Build history of the part. All positions in model axes, mm. Give positions to 0.01 mm unless a question says otherwise; leave off trailing zeros. Loops run counter-clockwise (first coordinate to the right, second up) from the corner with the lowest first, then second, coordinate; pieces in that order, holes last. Notation, with made-up numbers: M 88.25,12.5 L 123.25,12.5 A16 ccw 123.25,19.5 Z; hole C 0,66.25 d1. An arc over 180 degrees is marked long. Answer as a JSON object with one key per item and string values. Group by question number.
1. Slice it at A-A (x = 32.5). List the corners of the cut face in (y, z), then the cut area to 3 significant figures.
2. Mould opens along Z. For faces 1 (the face through (-10, 35, 20)), 2 (the face through (-0.462, 51.005, 19.493)), 3 (the face through (34.415, 35.496, 5.381)) say: released by +Z, released by -Z, zero draft, split by the parting line, or undercut.
3. Slice it at B-B (z = 11.25). Give the number of separate pieces and of enclosed holes in the cut face, then the cut area to 3 significant figures.
4. Drill centre lines: line 1 along X through (y, z) = (17, 11.25); line 2 along X through (y, z) = (7.5, 7.5); line 3 along Z through (x, y) = (-32.5, 27). Where is each one in solid material? Low to high. Write a range as [from, to].
5. Drop flat-ended pins along their axis: pin 1 Ø8 at (x, z) = (-70.5, 11) entering from -Y; pin 2 Ø3 at (x, z) = (-40, 7.5) entering from -Y; pin 3 Ø10 at (x, z) = (-55, 13) entering from -Y; pin 4 Ø6 at (x, z) = (32.5, 10) entering from -Y. Give the stop position or say it passes through.
from build123d import *

# Parameters (mm, degrees)
SKETCH1_W           = 86
SKETCH1_H           = 72
BOSS_EXTRUDE1_DEPTH = 20
SKETCH2_R           = 5
CUT_EXTRUDE1_DEPTH  = 87.214847909
FILLET1_R           = 0.5
FILLET2_R           = 0.5
SKETCH6_W           = 20
SKETCH6_H           = 72
BOSS_EXTRUDE2_DEPTH = 53
CAVITY1_OUTLINE_R   = 5
CAVITY1_DEPTH       = 20
CUT_EXTRUDE2_DEPTH  = 122.65525076


# Read off the part's stored shape, not the designer's step: Cavity1
with BuildPart() as part:
    # Sketch1 → Boss-Extrude1 (new body)
    with BuildSketch(Plane.XY):
        with Locations((0, 36)):
            Rectangle(SKETCH1_W, SKETCH1_H)
    extrude(amount=BOSS_EXTRUDE1_DEPTH)

    # Sketch2 → Cut-Extrude1 (cut, through all)
    with BuildSketch(Plane(origin=(0, 0, 0), x_dir=(1, 0, 0), z_dir=(0, 1, 0))):
        with Locations(Location((-32.5, -10, 0), (0, 0, 270))):
            Circle(SKETCH2_R)
        with Locations(Location((32.5, -10, 0), (0, 0, 90))):
            Circle(SKETCH2_R)
    extrude(amount=CUT_EXTRUDE1_DEPTH, mode=Mode.SUBTRACT)

    # Sketch4 → Cut-Revolve1 (revolve, cut)
    with BuildSketch(Plane(origin=(0, 72, 0), x_dir=(-1, 0, 0), z_dir=(0, 1, 0))):
        with BuildLine():
            Line((0, 0), (0, 20))
            Line((0, 20), (21, 20))
            Line((21, 20), (21, 18.5))
            Line((21, 18.5), (21.9089023, 18.5))
            ThreePointArc((21.9089023, 18.5), (23.5, 10), (21.9089023, 1.5))
            Line((21.9089023, 1.5), (21, 1.5))
            Line((21, 1.5), (21, 0))
            Line((21, 0), (0, 0))
        make_face()
    revolve(axis=Axis((0, 72, 0), (0, 0, 1)), mode=Mode.SUBTRACT)

    # Sketch5 → Cut-Revolve2 (revolve, cut)
    with BuildSketch(Plane(origin=(0, 48.5, 0), x_dir=(1, 0, 0), z_dir=(0, 1, 0))):
        with BuildLine():
            Line((0, -5), (0, -8))
            ThreePointArc((0, -8), (-1.5, -6.5), (0, -5))
        make_face()
    revolve(axis=Axis((0, 48.5, 0), (0, 0, 1)), mode=Mode.SUBTRACT)

    # Fillet1
    fillet1_edges = [part.edges().sort_by_distance(p)[0] for p in [
        (0, 50.0910977, 18.5),
        (0, 50.0910977, 1.5),
    ]]
    fillet(fillet1_edges, radius=FILLET1_R)

    # Fillet2
    fillet2_edges = [part.edges().sort_by_distance(p)[0] for p in [
        (0, 51, 18.5),
        (0, 51, 1.5),
    ]]
    fillet(fillet2_edges, radius=FILLET2_R)

    # Sketch6 → Boss-Extrude2 (add)
    with BuildSketch(Plane(origin=(-43, 0, 0), x_dir=(0, 0, -1), z_dir=(1, 0, 0))):
        with Locations((-10, 36)):
            Rectangle(SKETCH6_W, SKETCH6_H)
    extrude(amount=-BOSS_EXTRUDE2_DEPTH)

    # Cavity1 outline → Cavity1 (cut)
    with BuildSketch(Plane.XY):
        with Locations((-85.036371952, 40.687381171)):
            Circle(CAVITY1_OUTLINE_R)
    extrude(amount=CAVITY1_DEPTH, mode=Mode.SUBTRACT)

    # Sketch8 → Cut-Extrude2 (cut, through all)
    with BuildSketch(Plane.XY.offset(20)):
        with BuildLine():
            Line((-43.611081488, 0), (-43.611081488, -5.76813428))
            Line((-43.611081488, -5.76813428), (-107.878292828, -5.76813428))
            Line((-107.878292828, -5.76813428), (-107.878292828, 57.33150687))
            Line((-107.878292828, 57.33150687), (-107.878292828, 72))
            Line((-107.878292828, 72), (-43, 72))
            add(Edge.make_bspline(
                [(-95.73694265, 43.074623662), (-91.28097288, 63.04805315), (-43, 42.337327556), (-43, 72)],
                knots=[0, 0, 0, 0, 1, 1, 1, 1], degree=3))
            ThreePointArc((-95.73694265, 43.074623662), (-95.93403723, 41.888227318), (-96, 40.687381171))
            ThreePointArc((-96, 40.687381171), (-93.288759206, 33.469400526), (-86.495984658, 29.821348283))
            add(Edge.make_bspline(
                [(-86.495984658, 29.821348283), (-76.006838116, 28.412361974), (-38.381653368, 24.579008499), (-43.611081488, 22.17214242), (-43.611081488, 0)],
                knots=[0, 0, 0, 0, 0.346709448, 1, 1, 1, 1], degree=3))
        make_face()
    extrude(amount=-CUT_EXTRUDE2_DEPTH, mode=Mode.SUBTRACT)


solid = part.part
Established:
{
 "1": {"outline": "M 0,0 L 72,0 L 72,5 L 0,5 Z; M 0,15 L 72,15 L 72,20 L 0,20 Z", "area": "720 mm^2"},
 "2": {"face 1": "released by +Z", "face 2": "zero draft", "face 3": "undercut"},
 "3": {"separate pieces": "3", "enclosed holes": "1", "area": "5,260 mm^2"},
 "4": {"line 1": "x = [-43.3, -37.34], [-27.66, 27.66], [37.34, 43]", "line 2": "x = [-43.49, -36.83], [-28.17, 28.17], [36.83, 43]", "line 3": "z = [0, 5], [15, 20]"},
 "5": {"pin 1": "stops at y = 27.39", "pin 2": "stops at y = 0", "pin 3": "stops at y = 25.03", "pin 4": "passes through"}
}
